Check sheet for the modelled part. Datum: model origin and axes. Units: mm. Face numbers are marked on the shaded views. A direction names the side the tool comes from. Round coordinates to 2 decimals unless told otherwise and drop trailing zeros. Write each loop counter-clockwise with the first axis right and the second up, starting at its lowest first coordinate (ties: lowest second). Pieces come first, ordered by that corner, then holes.
Item 1: Depth check by flat-ended pin: pin 1 (8 mm diameter, centred on x = -8.5, y = 6, fed in from +Z). Enter the tip coordinate at first touch or a pass-through.
Item 2: Release check for a two-part mould opening along X. For the marked faces 3, 4, 5 and 6 record: pulls with the +X half, pulls with the -X half, needs draft (parallel to the pull), parting line crosses it, or undercut.
Item 3: Material ranges on line 1 along X through (y, z) = (-1.5, 7.25); line 2 along Z through (x, y) = (8.5, 8.5), recorded low to high.
Item 4: Set-up check for the marked faces 1 and 2: record each of +Z, -Z, +X, -X, +Y, -Y from which the full face is reachable in a straight line by a thin tool's end or side.
Item 5: Section check B-B, the plane y = 0.5. Record the cut outline in (x, z), plus the area to 3 significant figures.
Item 6: Section check D-D, the plane z = 2.75. Record the cut outline in (x, y).
Item 7: Section check A-A, the plane z = 18.5. Record the cut outline in (x, y), plus the area to 3 significant figures.
Item 8: Section check C-C, the plane y = 4.75. Record the cut outline in (x, z).
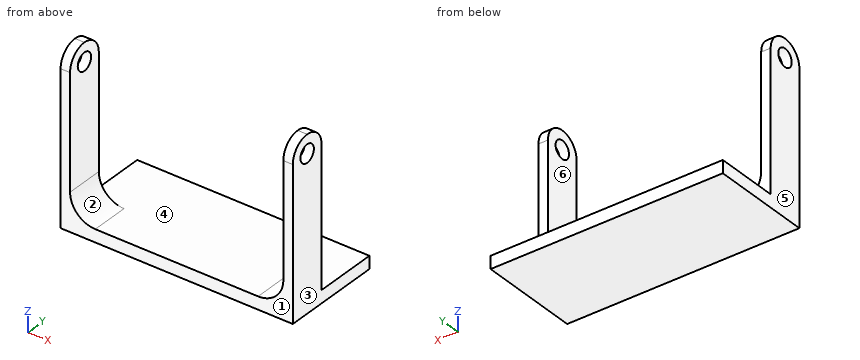
from build123d import *

# Parameters (mm, degrees)
SKETCH1_W           = 36.8
SKETCH1_H           = 6
BOSS_EXTRUDE1_DEPTH = 2
SKETCH2_W           = 1.5
SKETCH2_H           = 6
BOSS_EXTRUDE2_DEPTH = 25
SKETCH3_R           = 1.4
CUT_EXTRUDE1_DEPTH  = 46.741010046
FILLET1_R           = 3
SKETCH4_W           = 36.8
SKETCH4_H           = 2
BOSS_EXTRUDE3_DEPTH = 10
FILLET2_R           = 4


with BuildPart() as part:
    # Sketch1 → Boss-Extrude1 (new body)
    with BuildSketch(Plane.XY):
        Rectangle(SKETCH1_W, SKETCH1_H)
    extrude(amount=BOSS_EXTRUDE1_DEPTH)

    # Sketch2 → Boss-Extrude2 (add)
    with BuildSketch(Plane.XY.offset(2)):
        with Locations((-17.65, 0)):
            Rectangle(SKETCH2_W, SKETCH2_H)
        with Locations((17.65, 0)):
            Rectangle(SKETCH2_W, SKETCH2_H)
    extrude(amount=BOSS_EXTRUDE2_DEPTH)

    # Sketch3 → Cut-Extrude1 (cut, through all)
    with BuildSketch(Plane(origin=(18.4, 0, 0), x_dir=(0, 0, -1), z_dir=(1, 0, 0))):
        with Locations((-24.1, 0)):
            Circle(SKETCH3_R)
    extrude(amount=-CUT_EXTRUDE1_DEPTH, mode=Mode.SUBTRACT)

    # Fillet1
    fillet1_edges = [part.edges().sort_by_distance(p)[0] for p in [
        (-17.65, -3, 27),
        (17.65, -3, 27),
        (-17.65, 3, 27),
        (17.65, 3, 27),
    ]]
    fillet(fillet1_edges, radius=FILLET1_R - 0.0001)  # a hair under: the kernel refuses the full size

    # Sketch4 → Boss-Extrude3 (add)
    with BuildSketch(Plane(origin=(0, 3, 0), x_dir=(1, 0, 0), z_dir=(0, 1, 0))):
        with Locations((0, -1)):
            Rectangle(SKETCH4_W, SKETCH4_H)
    extrude(amount=BOSS_EXTRUDE3_DEPTH)

    # Fillet2
    fillet2_edges = [part.edges().sort_by_distance(p)[0] for p in [
        (16.9, 0, 2),
        (-16.9, 0, 2),
    ]]
    fillet(fillet2_edges, radius=FILLET2_R)


solid = part.part
Values found:
1. pin 1: stops at z = 2
2. face 3: pulls with the +X half
2. face 4: undercut
2. face 5: pulls with the -X half
2. face 6: undercut
3. line 1: x = -18.4 to -16.9, 16.9 to 18.4
3. line 2: z = 0 to 2
4. face 1: +Z, -Z, +X, -X, -Y
4. face 2: +Z, +Y, -Y
5. outline: (-18.4, 0) - (18.4, 0) - (18.4, 22.79) - (16.9, 22.79) - (16.9, 6) arc R4 cw to (12.9, 2) - (-12.9, 2) arc R4 cw to (-16.9, 6) - (-16.9, 22.79) - (-18.4, 22.79) - close; (-18.4, 25.41) - (-16.9, 25.41) - (-16.9, 26.96) - (-18.4, 26.96) - close; (16.9, 25.41) - (18.4, 25.41) - (18.4, 26.96) - (16.9, 26.96) - close
5. area: 147 mm2
6. outline: (-18.4, -3) - (-15.23, -3) - (-15.23, 3) - (-18.4, 3) - close; (15.23, -3) - (18.4, -3) - (18.4, 3) - (15.23, 3) - close
7. outline: (-18.4, -3) - (-16.9, -3) - (-16.9, 3) - (-18.4, 3) - close; (16.9, -3) - (18.4, -3) - (18.4, 3) - (16.9, 3) - close
7. area: 18.0 mm2
8. outline: (-18.4, 0) - (18.4, 0) - (18.4, 2) - (-18.4, 2) - close
